Design review of the part built by this model. Coordinates are the model's own, in mm. A direction names the side the tool comes from. Coordinates: 2 decimals unless noted, no trailing zeros. Loops run counter-clockwise (first coordinate to the right, second up) from the corner with the lowest first, then second, coordinate; pieces in that order, holes last. Notation, with made-up numbers: (44, 77.5) - (55, 77.5) arc R12 cw to (55, 92.5) - close; hole circle Ø7 at (81.25, 31.5). An arc over 180 degrees is marked (long way). One line per question, with ' | ' between items.
from build123d import *

# Parameters (mm, degrees)
SKETCH2_W                  = 38.1
SKETCH2_H                  = 38.1
SKETCH2_W_2                = 31.75
SKETCH2_H_2                = 31.75
BOSS_EXTRUDE1_DEPTH        = 1129.03
X_0_397_DIAMETER_HOLE1_D   = 10.0838
F_1_2_0_5_DIAMETER_HOLE1_D = 12.7


with BuildPart() as part:
    # Sketch2 → Boss-Extrude1 (new body)
    with BuildSketch(Plane.XY):
        with Locations((19.05, 19.05)):
            Rectangle(SKETCH2_W, SKETCH2_H)
        with Locations((19.05, 19.05)):
            Rectangle(SKETCH2_W_2, SKETCH2_H_2, mode=Mode.SUBTRACT)
    extrude(amount=BOSS_EXTRUDE1_DEPTH)

    # X (0.397) Diameter Hole1 (through all)
    with Locations(Plane.ZY):
        with Locations((19.05, 19.05), (361.95, 19.05)):
            Hole(X_0_397_DIAMETER_HOLE1_D / 2)

    # 1/2 (0.5) Diameter Hole1 (through all)
    with Locations(Plane.ZY):
        with Locations((1109.98, 19.05)):
            Hole(F_1_2_0_5_DIAMETER_HOLE1_D / 2)


solid = part.part
Q1. Take a section at A-A (x = 12.5). Give the boundary of the cut face in (y, z) (3 decimals), plus the area to 3 significant figures.
Returned:
outline: (0, 0) - (3.175, 0) - (3.175, 1129.03) - (0, 1129.03) - close; (34.925, 0) - (38.1, 0) - (38.1, 1129.03) - (34.925, 1129.03) - close | area: 7,170 mm²
Q2. Draft analysis for pull direction Y (two halves, no side actions). For faces 1 (the flat face through (3.175, 19, 557)), 2 (the flat face through (36, 19, 1129.03)), 3 (the flat face through (19, 0, 557)), state which applies: +Y half, -Y half, draft (parallel to the pull), parting line (faces both ways), or undercut.
Returned:
face 1: undercut | face 2: draft | face 3: -Y half
Q3. Tool access review of faces 4 (the flat face through (19, 3.175, 557)), 5 (the flat face through (0, 19, 557)): name each direction out of +Z, -Z, +X, -X, +Y, -Y from which nothing blocks a thin tool from reaching the whole face with its end or side.
Returned:
face 4: +Z, -Z | face 5: +Z, -Z, -X, +Y, -Y
Q4. Take a section at B-B (z = 84). Give the boundary of the cut face in (x, y) (3 decimals), plus the area to 3 significant figures.
Returned:
outline: (0, 0) - (38.1, 0) - (38.1, 38.1) - (0, 38.1) - close; hole (3.175, 3.175) - (34.925, 3.175) - (34.925, 34.925) - (3.175, 34.925) - close | area: 444 mm²
Q5. For pin 1 (10 mm diameter, centred on y = 19.05, z = 1109.98, fed in from -X) (3 decimals), flat-tipped, find the tip position at first contact; note if it passes through.
Returned:
pin 1: passes through
Q6. To check wall thickness, follow line 1 along Y through (x, z) = (35.8, 361.95); line 2 along Y through (x, z) = (5, 706) (3 decimals). State the ranges of each line that lie inside material, in increasing order.
Returned:
line 1: y = 0 to 14.01, 24.09 to 38.1 | line 2: y = 0 to 3.175, 34.925 to 38.1
